Can you work these out from the model? Positions are in its coordinate system, mm. A direction names the side the tool comes from. Coordinates: 2 decimals unless noted, no trailing zeros. Write each loop counter-clockwise with the first axis right and the second up, starting at its lowest first coordinate (ties: lowest second). Pieces come first, ordered by that corner, then holes. Notation, with made-up numbers: (9.25, 56) - (66.25, 56) arc R31 cw to (66.25, 84) - close; hole circle Ø3 at (6.5, -32). An arc over 180 degrees is marked (long way). Use one line per item in the form item = value. Start each with the question number.
(1) If we section it at D-D on z = 37.5: Please give me the cut outline in (x, y).
(2) On a 3-axis mill with a long thin cutter (end or side, diameter ignored), from which of +Z, -Z, +X, -X, +Y, -Y can I reach the whole of each face in a straight line? I mean faces 4 (the face through (-10, 14, 34)), 5 (the face through (0, -21, 38)), 6 (the face through (-13, 13, 36.6)). Say none if no direction works.
(3) For pin 1 Ø1 at (x, z) = (10, 31.5) entering from +Y; pin 2 Ø10 at (y, z) = (11, 16) entering from +X; pin 3 Ø9 at (x, y) = (15.2, -15.2) entering from -Z; pin 4 Ø3.5 at (x, y) = (-15.2, -15.2) entering from +Z, each with a flat end and sliding along its axis, tell me the tip position at first contact or that it passes through.
(4) If we section it at C-C on z = 22.5: Please give me the cut outline in (x, y).
(5) Thinking about a two-plate mould opening in X: for faces 1 (the face through (15.561, -12.476, 35.282)), 2 (the face through (-10, 10, 42)), 3 (the face through (-21, 0, 38)), which applies, pulls with the +X half, pulls with the -X half, needs draft (parallel to the pull), parting line crosses it, or undercut?
(6) If we section it at A-A on x = 0: Please give me the cut outline in (y, z), then the cut area to 3 significant figures.
(7) If I drill on probe 1 along Y at (x, z) = (-16, 36.5); probe 2 along Z at (x, y) = (10, 14.5); probe 3 along Y at (x, z) = (12.5, 14), over which ranges is the centre line in solid material (lowest first)? Write a range as from..to.
```python
from build123d import *

# Parameters (mm, degrees)
SKETCH1_R                                           = 16
BOSS_EXTRUDE1_DEPTH                                 = 42
SKETCH2_W                                           = 42
SKETCH2_H                                           = 42
BOSS_EXTRUDE2_DEPTH                                 = 8
CUT_EXTRUDE1_DEPTH                                  = 52.439284598
CBORE_FOR_M5_HEX_SOCKET_HEAD_CAP_SCREW1_D           = 5.5
CBORE_FOR_M5_HEX_SOCKET_HEAD_CAP_SCREW1_DEPTH       = 22
CBORE_FOR_M5_HEX_SOCKET_HEAD_CAP_SCREW1_CBORE_D     = 9.5
CBORE_FOR_M5_HEX_SOCKET_HEAD_CAP_SCREW1_CBORE_DEPTH = 5.4
CBORE_FOR_M5_HEX_SOCKET_HEAD_CAP_SCREW1_TIP         = 1.652366702
SKETCH8_R                                           = 10
CUT_EXTRUDE2_DEPTH                                  = 52.439284598
CHAMFER1_SIZE                                       = 1


with BuildPart() as part:
    # Sketch1 → Boss-Extrude1 (new body)
    with BuildSketch(Plane.XY):
        with Locations(Location((0, 0, 0), (0, 0, 180))):
            Circle(SKETCH1_R)
    extrude(amount=BOSS_EXTRUDE1_DEPTH)

    # Sketch2 → Boss-Extrude2 (add)
    with BuildSketch(Plane.XY.offset(42)):
        Rectangle(SKETCH2_W, SKETCH2_H)
    extrude(amount=-BOSS_EXTRUDE2_DEPTH)

    # Sketch4 → Cut-Extrude1 (cut, through all)
    with BuildSketch(Plane.XY.offset(42)):
        Polygon((-21, 21), (-21, 17.183766184), (-17.183766184, 21), align=None)
        Polygon((17.183766184, 21), (21, 21), (21, 17.183766184), align=None)
        Polygon((21, -21), (21, -17.183766184), (17.183766184, -21), align=None)
        Polygon((-17.183766184, -21), (-21, -21), (-21, -17.183766184), align=None)
    extrude(amount=-CUT_EXTRUDE1_DEPTH, mode=Mode.SUBTRACT)

    # CBORE for M5 Hex Socket Head Cap Screw1
    with Locations(Plane.XY.offset(42)):
        with Locations((-15.202795796, 15.202795796), (15.202795796, 15.202795796), (15.202795796, -15.202795796), (-15.202795796, -15.202795796)):
            CounterBoreHole(CBORE_FOR_M5_HEX_SOCKET_HEAD_CAP_SCREW1_D / 2, CBORE_FOR_M5_HEX_SOCKET_HEAD_CAP_SCREW1_CBORE_D / 2, CBORE_FOR_M5_HEX_SOCKET_HEAD_CAP_SCREW1_CBORE_DEPTH, depth=CBORE_FOR_M5_HEX_SOCKET_HEAD_CAP_SCREW1_DEPTH)
            with Locations((0, 0, -(CBORE_FOR_M5_HEX_SOCKET_HEAD_CAP_SCREW1_DEPTH + CBORE_FOR_M5_HEX_SOCKET_HEAD_CAP_SCREW1_TIP / 2))):  # 118° drill point
                Cone(0, CBORE_FOR_M5_HEX_SOCKET_HEAD_CAP_SCREW1_D / 2, CBORE_FOR_M5_HEX_SOCKET_HEAD_CAP_SCREW1_TIP, mode=Mode.SUBTRACT)

    # Sketch8 → Cut-Extrude2 (cut, through all)
    with BuildSketch(Plane.XY.offset(42)):
        Circle(SKETCH8_R)
    extrude(amount=-CUT_EXTRUDE2_DEPTH, mode=Mode.SUBTRACT)

    # Chamfer1
    chamfer1_edges = [part.edges().sort_by_distance(p)[0] for p in [
        (-10, 0, 42),
        (16, 0, 0),
    ]]
    chamfer(chamfer1_edges, length=CHAMFER1_SIZE)


solid = part.part
```
Reported:
q1.outline = (-21, -17.18) - (-17.18, -21) - (17.18, -21) - (21, -17.18) - (21, 17.18) - (17.18, 21) - (-17.18, 21) - (-21, 17.18) - close; hole circle Ø9.5 at (-15.2, -15.2); hole circle Ø9.5 at (-15.2, 15.2); hole circle Ø20 at (0, 0); hole circle Ø9.5 at (15.2, -15.2); hole circle Ø9.5 at (15.2, 15.2)
q2.face_4 = -Z
q2.face_5 = +Z, -Z, +X, -X, -Y
q2.face_6 = +Z
q3.pin_1 = 12.87
q3.pin_2 = 14.83
q3.pin_3 = 34
q3.pin_4 = through
q4.outline = circle Ø32 at (0, 0); hole circle Ø20 at (0, 0)
q5.face_1 = undercut
q5.face_2 = needs draft
q5.face_3 = pulls with the -X half
q6.outline = (-21, 34) - (-16, 34) - (-16, 1) - (-15, 0) - (-10, 0) - (-10, 41) - (-11, 42) - (-21, 42) - close; (10, 0) - (15, 0) - (16, 1) - (16, 34) - (21, 34) - (21, 42) - (11, 42) - (10, 41) - close
q6.area = 582 mm2
q7.probe_1 = -21..-17.83, -12.57..12.57, 17.83..21
q7.probe_2 = 34..42
q7.probe_3 = -9.99..9.99
